Could you check a few things on this model? Use its own coordinates, in mm. Face numbers are marked on the shaded views. A direction names the side the tool comes from. Give positions to 0.01 mm unless a question says otherwise; leave off trailing zeros. Loops run counter-clockwise (first coordinate to the right, second up) from the corner with the lowest first, then second, coordinate; pieces in that order, holes last. Notation, with made-up numbers: (-3, 80.25) - (32, 80.25) arc R16 ccw to (32, 104.25) - close; hole circle Ø2 at (75, -16). An arc over 180 degrees is marked (long way). Answer in a Markdown table with one row per item. Add a question column.
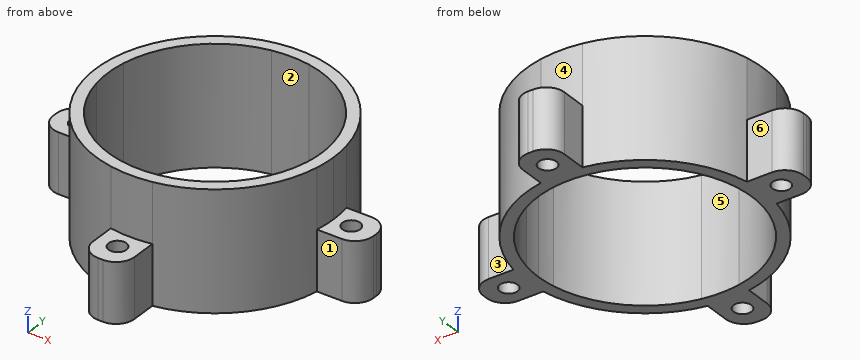
```python
from build123d import *

# Parameters (mm, degrees)
F1_DEPTH = 20
F2_T     = -2
F3_DEPTH = 10
F4_R     = 3.1
F5_D     = 3


with BuildPart() as f1:
    # F0 (on Top) → F1 (new body)
    with BuildSketch(Plane.XY):
        with BuildLine():
            ThreePointArc((19.691369, -3.5), (19.922693, -1.756791), (20, 0))
            ThreePointArc((20, 0), (19.922693, 1.756791), (19.691369, 3.5))
            ThreePointArc((19.691369, 3.5), (14.142136, 14.142136), (3.5, 19.691369))
            ThreePointArc((3.5, 19.691369), (0, 20), (-3.5, 19.691369))
            ThreePointArc((-3.5, 19.691369), (-14.142136, 14.142136), (-19.691369, 3.5))
            ThreePointArc((-19.691369, 3.5), (-20, 0), (-19.691369, -3.5))
            ThreePointArc((-19.691369, -3.5), (-14.142136, -14.142136), (-3.5, -19.691369))
            ThreePointArc((-3.5, -19.691369), (0, -20), (3.5, -19.691369))
            ThreePointArc((3.5, -19.691369), (14.142136, -14.142136), (19.691369, -3.5))
        make_face()
    extrude(amount=F1_DEPTH)

    # F2
    f2_openings = [f1.faces().sort_by_distance(p)[0] for p in [
        (0, 0, 20),
        (0, 0, 0),
    ]]
    offset(amount=F2_T, openings=f2_openings)

    # F0 (on Top) → F3 (join)
    with BuildSketch(Plane.XY):
        with BuildLine():
            ThreePointArc((-19.691369, -3.5), (-20, 0), (-19.691369, 3.5))
            Line((-19.691369, 3.5), (-27, 3.5))
            Line((-27, 3.5), (-27, -3.5))
            Line((-27, -3.5), (-19.691369, -3.5))
        make_face()
        with BuildLine():
            ThreePointArc((-3.5, 19.691369), (0, 20), (3.5, 19.691369))
            Line((3.5, 19.691369), (3.5, 27))
            Line((3.5, 27), (-3.5, 27))
            Line((-3.5, 27), (-3.5, 19.691369))
        make_face()
        with BuildLine():
            ThreePointArc((19.691369, 3.5), (19.922693, 1.756791), (20, 0))
            ThreePointArc((20, 0), (19.922693, -1.756791), (19.691369, -3.5))
            Line((19.691369, -3.5), (27, -3.5))
            Line((27, -3.5), (27, 3.5))
            Line((27, 3.5), (19.691369, 3.5))
        make_face()
        with BuildLine():
            Line((3.5, -27), (3.5, -19.691369))
            ThreePointArc((3.5, -19.691369), (0, -20), (-3.5, -19.691369))
            Line((-3.5, -19.691369), (-3.5, -27))
            Line((-3.5, -27), (3.5, -27))
        make_face()
    extrude(amount=F3_DEPTH)

    # F4
    f4_edges = [f1.edges().sort_by_distance(p)[0] for p in [
        (27, 3.5, 5),
        (27, -3.5, 5),
        (3.5, 27, 5),
        (3.5, -27, 5),
        (-27, -3.5, 5),
        (-3.5, -27, 5),
        (-27, 3.5, 5),
        (-3.5, 27, 5),
    ]]
    fillet(f4_edges, radius=F4_R)

    # F5 (through all)
    with Locations(Plane(origin=(0, 0, 0), x_dir=(1, 0, 0), z_dir=(0, 0, -1))):
        with Locations((23, 0), (0, -23), (-23, 0), (0, 23)):
            Hole(F5_D / 2)


solid = f1.part
```
(1) I want a section at C-C on z = 5.5. State how many separate pieces and enclosed holes the cut face has, then the cut area to 3 significant figures.
(2) For pin 1 Ø1.3 at (y, z) = (-22.5, 4) entering from +X; pin 2 Ø12 at (y, z) = (-14.5, 9) entering from -X; pin 3 Ø3.5 at (y, z) = (-23, 7.5) entering from -X; pin 4 Ø1 at (x, y) = (16.5, -15) entering from +Z, each with a flat end and sliding along its axis, tell me the tip position at first contact or that it passes through.
(3) Please list where these lines run through material, in increasing order: line 1 (X direction, y = -23, z = 5.5); line 2 (X direction, y = -14, z = 10).
(4) We'd pull the mould along X, two halves only. Please class the marked faces 4, 5 and 6: pulls with the +X half, pulls with the -X half, needs draft (parallel to the pull), parting line crosses it, or undercut.
(5) On a 3-axis mill with a long thin cutter (end or side, diameter ignored), from which of +Z, -Z, +X, -X, +Y, -Y can I reach the whole of each face in a straight line? I mean the marked faces 1, 2 and 3. Say none if no direction works.
(6) I want a section at A-A on x = 23. Please give me the cut outline in (y, z).
Reported:
| question | item | result |
|---|---|---|
| 1 | separate pieces | 1 |
| 1 | enclosed holes | 5 |
| 1 | area | 393 mm² |
| 2 | pin 1 | x = 3.5 |
| 2 | pin 2 | x = -18.1 |
| 2 | pin 3 | x = -3.5 |
| 2 | pin 4 | through |
| 3 | line 1 | -3.5 to -1.5, 1.5 to 3.5 |
| 3 | line 2 | -14.28 to -11.31, 11.31 to 14.28 |
| 4 | face 4 | parting line crosses it |
| 4 | face 5 | undercut |
| 4 | face 6 | needs draft |
| 5 | face 1 | +Z, -Z, +X, -Y |
| 5 | face 2 | +Z, -Z |
| 5 | face 3 | +Z, -Z, +X, +Y |
| 6 | outline | (-3.5, 0) - (-1.5, 0) - (-1.5, 10) - (-3.5, 10) - close; (1.5, 0) - (3.5, 0) - (3.5, 10) - (1.5, 10) - close |
